Read the model definition and answer for the solid it produces. Units are mm, in the model's axes. Face numbers are marked on the shaded views. Give positions to 0.01 mm unless a question says otherwise; leave off trailing zeros. Write each loop counter-clockwise with the first axis right and the second up, starting at its lowest first coordinate (ties: lowest second). Pieces come first, ordered by that corner, then holes. Notation, with made-up numbers: (-24, 44) - (-10, 44) arc R32 cw to (-10, 70) - close; hole circle Ø8 at (-26, -32). An arc over 180 degrees is marked (long way). Answer as CSV lines item,"result".
```python
from build123d import *

# Parameters (mm, degrees)
ESBO_O2_R = 15
CASCA1_T  = -2


with BuildPart() as part:
    # Varredura1: sweep along a path in Esboço1
    with BuildLine(Plane.XY) as varredura1_path:
        Line((0, 0), (0, 110))
        ThreePointArc((0, 110), (11.715728753, 138.284271247), (40, 150))
        Line((40, 150), (150, 150))
    # Esboço2 → Varredura1 (sweep)
    with BuildSketch(Plane(origin=(0, 0, 0), x_dir=(1, 0, 0), z_dir=(0, 1, 0))):
        Circle(ESBO_O2_R)
    sweep(path=varredura1_path.line)

    # Casca1
    casca1_openings = [part.faces().sort_by_distance(p)[0] for p in [
        (150, 150, 0),
        (0, 0, 0),
    ]]
    offset(amount=CASCA1_T, openings=casca1_openings, kind=Kind.INTERSECTION)


solid = part.part
```
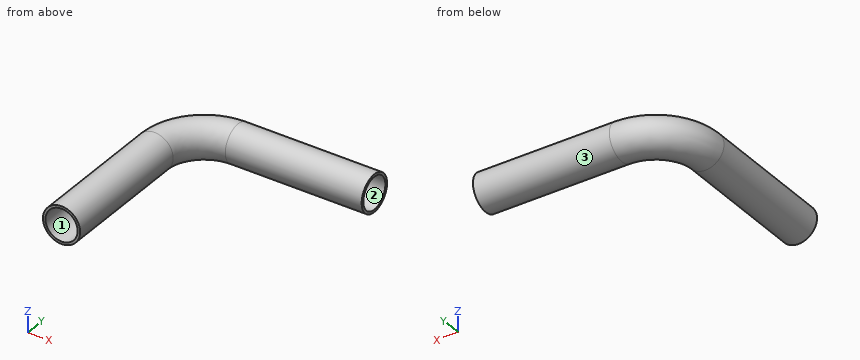
(1) A cutting plane is placed at D-D (z = -9). Write down the section's boundary in (x, y), and give its area (3 significant figures).
Worked out:
outline,"(-12, 0) - (-9.38, 0) - (-9.38, 110) arc R49.38 cw to (40, 159.38) - (150, 159.38) - (150, 162) - (40, 162) arc R52 ccw to (-12, 110) - close; (9.38, 0) - (12, 0) - (12, 110) arc R28 cw to (40, 138) - (150, 138) - (150, 140.62) - (40, 140.62) arc R30.62 ccw to (9.38, 110) - close"
area,"1,480 mm^2"
(2) A cutting plane is placed at C-C (y = 98). Write down the section's boundary in (x, z).
Worked out:
outline,"circle Ø30 at (0, 0); hole circle Ø26 at (0, 0)"
(3) Find the intervals of material crossed by L1, parallel to Y at x = 65, z = 0; L2, parallel to Z at x = 0, y = 74.5, in increasing order.
Worked out:
L1,"y = 135 to 137, 163 to 165"
L2,"z = -15 to -13, 13 to 15"
(4) Each of these flat-tipped pins is pushed along its axis until it touches: P1, Ø3, axis at x = 74.5, z = -5.5, coming from the +Y side; P2, Ø1.5, axis at x = 120, z = 1, coming from the -Y side; P3, Ø6, axis at x = 9, z = 0, coming from the +Y side. Where does it stop, or does it pass through?
Worked out:
P1,"stops at y = 164.46"
P2,"stops at y = 135"
P3,"stops at y = 157.34"
(5) A cutting plane is placed at A-A (z = 0). Write down the section's boundary in (x, y), and give its area (3 significant figures).
Worked out:
outline,"(-15, 0) - (-13, 0) - (-13, 110) arc R53 cw to (40, 163) - (150, 163) - (150, 165) - (40, 165) arc R55 ccw to (-15, 110) - close; (13, 0) - (15, 0) - (15, 110) arc R25 cw to (40, 135) - (150, 135) - (150, 137) - (40, 137) arc R27 ccw to (13, 110) - close"
area,"1,130 mm^2"
(6) A cutting plane is placed at B-B (x = 126.5). Write down the section's boundary in (y, z), and give its area (3 significant figures).
Worked out:
outline,"circle Ø30 at (150, 0); hole circle Ø26 at (150, 0)"
area,"176 mm^2"
(7) The mould has two halves that part along Z. Classify the marked faces 1, 2 and 3: +Z half, -Z half, draft (parallel to the pull), parting line (faces both ways), or undercut.
Worked out:
face 1,"undercut"
face 2,"undercut"
face 3,"parting line"
